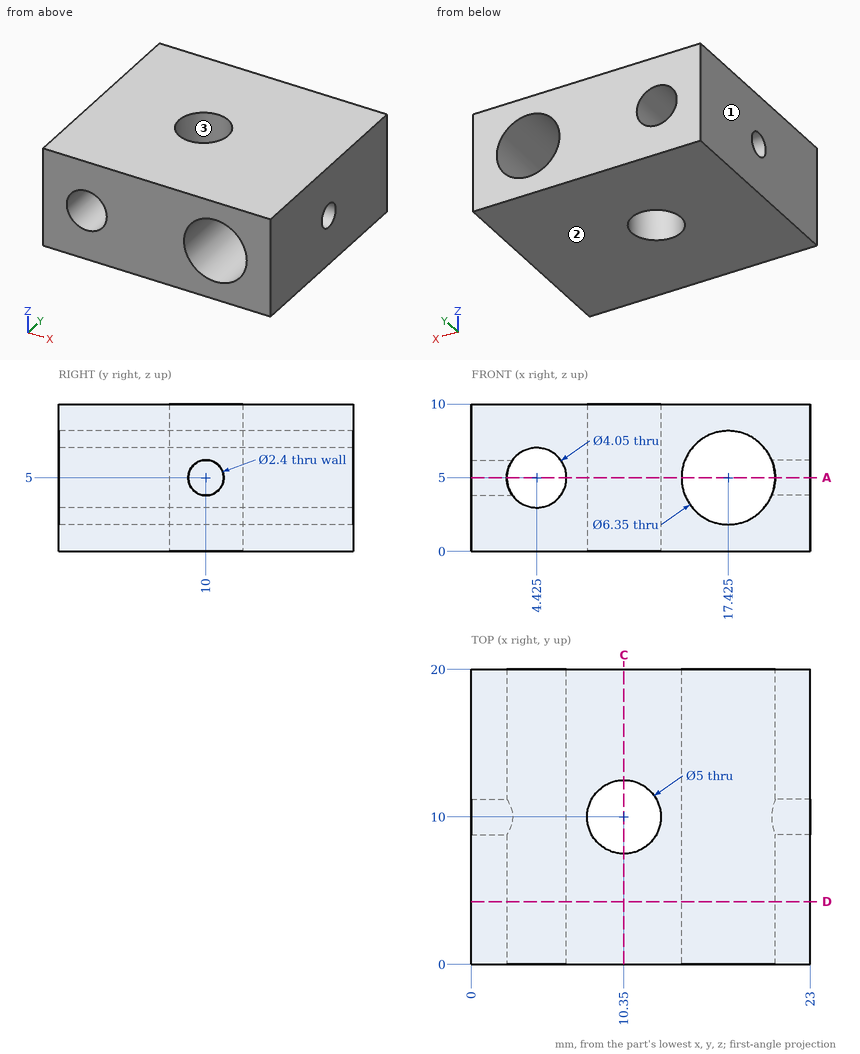
Answer from the drawing. Dimensions are ordinates in mm from the lowest x, y and z of the part. Round coordinates to 2 decimals unless told otherwise and drop trailing zeros. Write each loop counter-clockwise with the first axis right and the second up, starting at its lowest first coordinate (ties: lowest second). Pieces come first, ordered by that corner, then holes. Notation, with made-up numbers: (50, -30) -> (102, -30) arc R10 ccw to (102, -26) -> close; hole circle Ø10 at (-24.75, 60). An arc over 180 degrees is marked (long way). Write each question's results on one line, items separated by ' | '.
1) Flat-ended cylindrical pins translate along their axes: pin 1 (3 mm diameter, centred on x = 10.35, y = 10, fed in from -Z); pin 2 (1.9 mm diameter, centred on y = 10, z = 5, fed in from +X). Find the tip coordinate at first contact, or state that the pin passes through.
Findings:
pin 1: passes through | pin 2: stops at x = 14.4
2) The part is cut by section A-A (z = 5). Write down the section's boundary in (x, y).
Findings:
outline: (0, 0) -> (2.4, 0) -> (2.4, 8.8) -> (0, 8.8) -> close; (0, 11.2) -> (2.4, 11.2) -> (2.4, 20) -> (0, 20) -> close; (6.45, 0) -> (14.25, 0) -> (14.25, 20) -> (6.45, 20) -> close; (20.6, 0) -> (23, 0) -> (23, 8.8) -> (20.6, 8.8) -> close; (20.6, 11.2) -> (23, 11.2) -> (23, 20) -> (20.6, 20) -> close; hole circle Ø5 at (10.35, 10)
3) The part is cut by section D-D (y = 4.25). Write down the section's boundary in (x, z) (3 decimals), and give its area (3 significant figures).
Findings:
outline: (0, 0) -> (23, 0) -> (23, 10) -> (0, 10) -> close; hole circle Ø4.05 at (4.425, 5); hole circle Ø6.35 at (17.425, 5) | area: 185 mm²
4) The part is cut by section C-C (x = 10.35). Write down the section's boundary in (y, z), and give its area (3 significant figures).
Findings:
outline: (0, 0) -> (7.5, 0) -> (7.5, 10) -> (0, 10) -> close; (12.5, 0) -> (20, 0) -> (20, 10) -> (12.5, 10) -> close | area: 150 mm²
5) For a pull along X with two mould halves and no side action, classify the marked faces 1, 2 and 3 as +X half, -X half, draft (parallel to the pull), parting line (faces both ways), or undercut.
Findings:
face 1: -X half | face 2: draft | face 3: undercut
6) Consider line 1 along Z through (x, y) = (4.5, 5); line 2 along Y through (x, z) = (10.35, 4.5); line 3 along Z through (x, y) = (1.8, 10). Determine where each line is inside the solid, lowest interval first. Write a range as [from, to].
Findings:
line 1: z = [0, 2.98], [7.02, 10] | line 2: y = [0, 7.5], [12.5, 20] | line 3: z = [0, 3.8], [6.2, 10]
